Read the model definition and answer for the solid it produces. Units are mm, in the model's axes. A direction names the side the tool comes from. Round coordinates to 2 decimals unless told otherwise and drop trailing zeros. Loops run counter-clockwise (first coordinate to the right, second up) from the corner with the lowest first, then second, coordinate; pieces in that order, holes last. Notation, with made-up numbers: M -30.5,66 L 13.5,66 A11 cw 13.5,81 Z; hole C 68,19.25 d9. An arc over 180 degrees is marked long. Write each question's results on one line, items separated by ' | '.
```python
from build123d import *

# Parameters (mm, degrees)
F0_W     = 508
F0_H     = 254
F1_DEPTH = 19.05
F2_W     = 19.05
F2_H     = 38.1
F3_DEPTH = 19.05
F4_W     = 508
F4_H     = 19.05
F5_DEPTH = 19.05


with BuildPart() as f1:
    # F0 (on Top) → F1 (new body)
    with BuildSketch(Plane.XY):
        with Locations((-19.604288, 68.676595)):
            Rectangle(F0_W, F0_H)
    extrude(amount=F1_DEPTH)

    # F2 (on face) → F3 (cut)
    with BuildSketch(Plane.XY.offset(19.05)):
        with Locations((-264.079288, 119.476595)):
            Rectangle(F2_W, F2_H)
        with Locations((-264.079288, 17.876595)):
            Rectangle(F2_W, F2_H)
        with Locations((224.870712, 119.476595)):
            Rectangle(F2_W, F2_H)
        with Locations((224.870712, 17.876595)):
            Rectangle(F2_W, F2_H)
    extrude(amount=-F3_DEPTH, mode=Mode.SUBTRACT)

    # F4 (on face) → F5 (join)
    with BuildSketch(Plane.XZ.offset(58.323405)):
        with Locations((-19.604288, 9.525)):
            Rectangle(F4_W, F4_H)
    extrude(amount=F5_DEPTH)


solid = f1.part
```
1. Determine the mould class of faces 1 (the face through (225, 36.927, 10)), 2 (the face through (234.396, 167, 9)), 3 (the face through (-23, -77.373, 10)) for opening direction Y: released by +Y, released by -Y, zero draft, split by the parting line, or undercut.
Completed:
face 1: undercut | face 2: zero draft | face 3: released by -Y
2. Given P1, Ø5.5, axis at y = 125, z = 9.5, coming from the -X side; P2, Ø5.5, axis at y = 113, z = 10.5, coming from the +X side, each flat-ended and moving along its own axis, determine where each tip first touches the part or whether it passes through.
Completed:
P1: stops at x = -254.55 | P2: stops at x = 215.35
3. Which of the six approach directions +Z, -Z, +X, -X, +Y, -Y give full straight-line access (tool end or side, diameter ignored) to faces 4 (the face through (225, -1.173, 10)), 5 (the face through (-23, 195.677, 9)), 6 (the face through (-264, 36.927, 10))?
Completed:
face 4: +Z, -Z, +X | face 5: +Z, -Z, +X, -X, +Y | face 6: +Z, -Z, -X
4. Find section B-B, the plane y = 129. Give the vertices of the cut face in (x, z).
Completed:
outline: M -254.55,0 L 215.35,0 L 215.35,19.05 L -254.55,19.05 Z
5. Find the intervals of material crossed by L1, parallel to X at y = 23.5, z = 1.75, in increasing order.
Completed:
L1: x = -254.55 to 215.35
6. Find section A-A, the plane z = 3.5. Give the vertices of the cut face in (x, y).
Completed:
outline: M -273.6,-77.37 L 234.4,-77.37 L 234.4,-1.17 L 215.35,-1.17 L 215.35,36.93 L 234.4,36.93 L 234.4,100.43 L 215.35,100.43 L 215.35,138.53 L 234.4,138.53 L 234.4,195.68 L -273.6,195.68 L -273.6,138.53 L -254.55,138.53 L -254.55,100.43 L -273.6,100.43 L -273.6,36.93 L -254.55,36.93 L -254.55,-1.17 L -273.6,-1.17 Z
